Here's how the part is built. I have some questions about the finished solid (model axes, mm). A direction names the side the tool comes from. Round coordinates to 2 decimals unless told otherwise and drop trailing zeros. Order: outer loops, then holes, each group sorted by start corner. A loop starts at its lowest first (then second) coordinate and runs counter-clockwise, first axis right, second up. Notation, with made-up numbers: (64.5, 75) -> (89.5, 75) arc R20 cw to (89.5, 81) -> close; hole circle Ø5 at (-30.5, -15.5). An arc over 180 degrees is marked (long way). Use a Markdown table: item, result. Add a question column.
from build123d import *

# Parameters (mm, degrees)
F0_W     = 190.5
F0_H     = 127
F0_R     = 7.14375
F1_DEPTH = 11.176
F2_W     = 6.35
F2_H     = 60.325
F2_H_2   = 6.35
F2_W_2   = 92.075
F3_DEPTH = 152.4
F4_W     = 190.5
F4_H     = 127
F5_DEPTH = 11.176
F7_DEPTH = 25.4


with BuildPart() as f1:
    # F0 (on Top) → F1 (new body)
    with BuildSketch(Plane.XY):
        Rectangle(F0_W, F0_H)
        with Locations((-79.375, -47.752)):
            Circle(F0_R, mode=Mode.SUBTRACT)
        with Locations((79.375, -47.752)):
            Circle(F0_R, mode=Mode.SUBTRACT)
        with Locations((-79.375, 47.752)):
            Circle(F0_R, mode=Mode.SUBTRACT)
        with Locations((79.375, 47.752)):
            Circle(F0_R, mode=Mode.SUBTRACT)
    extrude(amount=-F1_DEPTH)

    # F2 (on face) → F3 (join)
    with BuildSketch(Plane.XY):
        with Locations((0, 33.3375)):
            Rectangle(F2_W, F2_H)
        Rectangle(F2_W, F2_H_2)
        with Locations((-49.2125, 0)):
            Rectangle(F2_W_2, F2_H_2)
        with Locations((49.2125, 0)):
            Rectangle(F2_W_2, F2_H_2)
        with Locations((0, -33.3375)):
            Rectangle(F2_W, F2_H)
    extrude(amount=F3_DEPTH)

    # F4 (on face) → F5 (join)
    with BuildSketch(Plane.XY.offset(152.4)):
        Rectangle(F4_W, F4_H)
    extrude(amount=F5_DEPTH)

    # F6 (on face) → F7 (cut)
    with BuildSketch(Plane.XY.offset(163.576)):
        with BuildLine():
            ThreePointArc((-57.94375, -30.226), (-63.5, -24.66975), (-69.05625, -30.226))
            Line((-69.05625, -30.226), (-69.05625, -45.974))
            ThreePointArc((-69.05625, -45.974), (-63.5, -51.53025), (-57.94375, -45.974))
            Line((-57.94375, -45.974), (-57.94375, -30.226))
        make_face()
        with BuildLine():
            Line((69.05625, -45.974), (69.05625, -30.226))
            ThreePointArc((69.05625, -30.226), (63.5, -24.66975), (57.94375, -30.226))
            Line((57.94375, -30.226), (57.94375, -45.974))
            ThreePointArc((57.94375, -45.974), (63.5, -51.53025), (69.05625, -45.974))
        make_face()
        with BuildLine():
            Line((-69.05625, 45.974), (-69.05625, 30.226))
            ThreePointArc((-69.05625, 30.226), (-63.5, 24.66975), (-57.94375, 30.226))
            Line((-57.94375, 30.226), (-57.94375, 45.974))
            ThreePointArc((-57.94375, 45.974), (-63.5, 51.53025), (-69.05625, 45.974))
        make_face()
        with BuildLine():
            ThreePointArc((57.94375, 30.226), (63.5, 24.66975), (69.05625, 30.226))
            Line((69.05625, 30.226), (69.05625, 45.974))
            ThreePointArc((69.05625, 45.974), (63.5, 51.53025), (57.94375, 45.974))
            Line((57.94375, 45.974), (57.94375, 30.226))
        make_face()
    extrude(amount=-F7_DEPTH, mode=Mode.SUBTRACT)


solid = f1.part
(1) I'm going to push flat-ended pins straight in: P1, Ø4, axis at x = 16.5, z = 22.5, coming from the -Y side (3 decimals); P2, Ø4, axis at y = -37, z = 129, coming from the +X side (3 decimals); P3, Ø5, axis at y = -13.5, z = 102, coming from the -X side (3 decimals). Where does each tip first touch, or does it pass through?
(2) I want a section at D-D on y = -15.5. List the corners of the cut face in (x, z) for me (3 decimals), and give its area (3 significant figures).
(3) I want a section at A-A on x = 63.5. List the corners of the cut face in (y, z) for me (3 decimals), and give its area (3 significant figures).
(4) I want a section at B-B on y = 38. List the corners of the cut face in (x, z) for me (3 decimals).
(5) I want a section at C-C on z = 107. List the corners of the cut face in (x, y) for me (3 decimals).
(6) On a 3-axis mill with a long thin cutter (end or side, diameter ignored), from which of +Z, -Z, +X, -X, +Y, -Y can I reach the whole of each face in a straight line? I mean faces 4 (the flat face through (49, -33, 152.4)), 5 (the cylindrical face through (-80.924, -54.726, -5.51)), 6 (the cylindrical face through (63.62, 51.53, 158.07)). Say none if no direction works.
(7) If we mould it in two halves opening along X, with no side actions, what happens to faces 1 (the flat face through (-3.175, -34, 75)), 2 (the flat face through (-1, 1, 163.576)), 3 (the flat face through (-69.056, -38, 158))? For each: pulls with the +X half, pulls with the -X half, needs draft (parallel to the pull), parting line crosses it, or undercut.
(8) Please list where these lines run through material, in increasing order: probe 1 along Z at (x, y) = (-25, -38); probe 2 along Y at (x, z) = (83, 1.5) (3 decimals). Write a range as from..to.
Output:
| question | item | result |
|---|---|---|
| 1 | P1 | y = -3.175 |
| 1 | P2 | x = 3.175 |
| 1 | P3 | x = -3.175 |
| 2 | outline | (-95.25, -11.176) -> (95.25, -11.176) -> (95.25, 0) -> (3.175, 0) -> (3.175, 152.4) -> (95.25, 152.4) -> (95.25, 163.576) -> (-95.25, 163.576) -> (-95.25, 152.4) -> (-3.175, 152.4) -> (-3.175, 0) -> (-95.25, 0) -> close |
| 2 | area | 5,230 mm² |
| 3 | outline | (-63.5, -11.176) -> (63.5, -11.176) -> (63.5, 0) -> (3.175, 0) -> (3.175, 152.4) -> (24.67, 152.4) -> (24.67, 163.576) -> (-24.67, 163.576) -> (-24.67, 152.4) -> (-3.175, 152.4) -> (-3.175, 0) -> (-63.5, 0) -> close; (-63.5, 152.4) -> (-51.53, 152.4) -> (-51.53, 163.576) -> (-63.5, 163.576) -> close; (51.53, 152.4) -> (63.5, 152.4) -> (63.5, 163.576) -> (51.53, 163.576) -> close |
| 3 | area | 3,210 mm² |
| 4 | outline | (-95.25, -11.176) -> (95.25, -11.176) -> (95.25, 0) -> (3.175, 0) -> (3.175, 152.4) -> (57.944, 152.4) -> (57.944, 163.576) -> (-57.944, 163.576) -> (-57.944, 152.4) -> (-3.175, 152.4) -> (-3.175, 0) -> (-95.25, 0) -> close; (-95.25, 152.4) -> (-69.056, 152.4) -> (-69.056, 163.576) -> (-95.25, 163.576) -> close; (69.056, 152.4) -> (95.25, 152.4) -> (95.25, 163.576) -> (69.056, 163.576) -> close |
| 5 | outline | (-95.25, -3.175) -> (-3.175, -3.175) -> (-3.175, -63.5) -> (3.175, -63.5) -> (3.175, -3.175) -> (95.25, -3.175) -> (95.25, 3.175) -> (3.175, 3.175) -> (3.175, 63.5) -> (-3.175, 63.5) -> (-3.175, 3.175) -> (-95.25, 3.175) -> close |
| 6 | face 4 | +X, -Y |
| 6 | face 5 | -Z |
| 6 | face 6 | +Z |
| 7 | face 1 | pulls with the -X half |
| 7 | face 2 | needs draft |
| 7 | face 3 | undercut |
| 8 | probe 1 | -11.18..0, 152.4..163.58 |
| 8 | probe 2 | -3.175..3.175 |
